Here's the drawing with two shaded views (mm, measured from the low corner). I have some questions. Round coordinates to 2 decimals unless told otherwise and drop trailing zeros. Write each loop counter-clockwise with the first axis right and the second up, starting at its lowest first coordinate (ties: lowest second). Pieces come first, ordered by that corner, then holes. Notation, with made-up numbers: M -14.5,-26.75 L -5.5,-26.75 A24 ccw -5.5,-11.75 Z; hole C 48,80 d5. An arc over 180 degrees is marked long. Use one line per item in the form item = value. Start each with the question number.
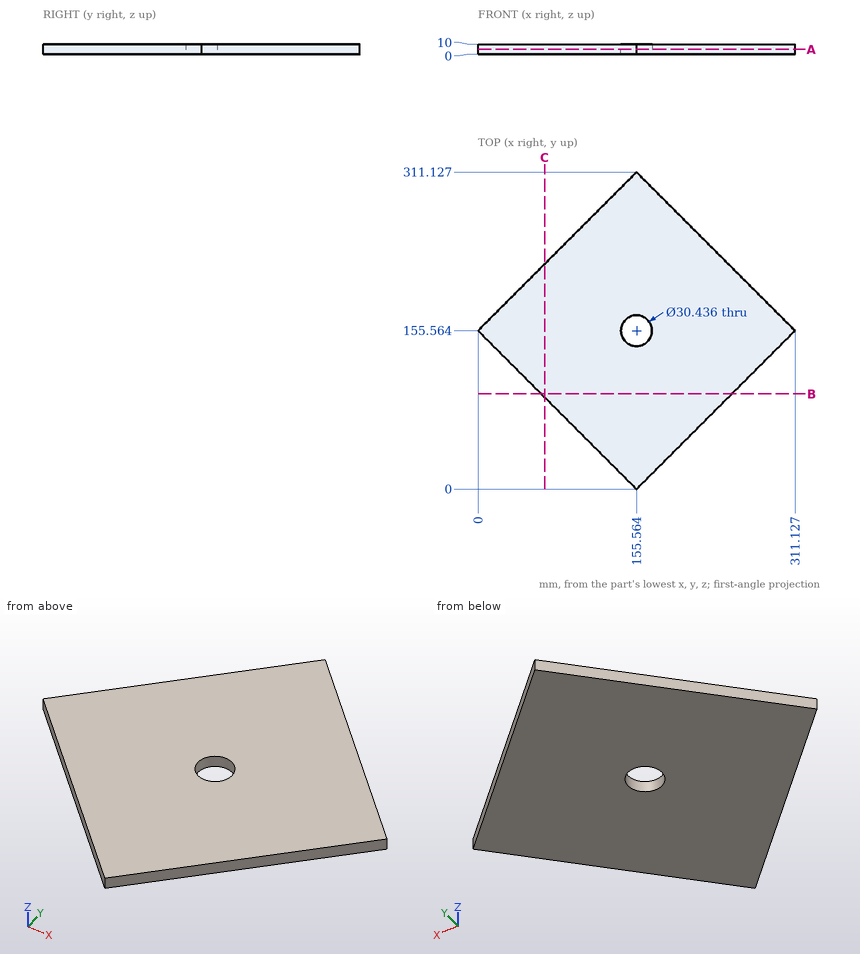
1. Please list where these lines run through material, in increasing order: line 1 along Y through (x, z) = (153.5, 7.75) (1 decimal); line 2 along Y through (x, z) = (168, 3.5) (1 decimal); line 3 along X through (y, z) = (110, 8.75) (1 decimal).
2. If we section it at B-B (y = 93.5): List the corners of the cut face in (x, z) for me.
3. If we section it at A-A (z = 4.75): List the corners of the cut face in (x, y) for me (1 decimal), and give its area (3 significant figures).
4. If we section it at C-C (x = 65.5): List the corners of the cut face in (y, z) for me, and give its area (3 significant figures).
5. Will these pins go through, and if not, where does the flat tip stop? pin 1 (6 mm diameter, centred on x = 260, z = 4.5, fed in from +Y); pin 2 (6 mm diameter, centred on y = 191.5, z = 3, fed in from -X) (1 decimal); pin 3 (1 mm diameter, centred on y = 90, z = 7, fed in from -X) (1 decimal).
Model answer:
q1.line_1 = 2.1 to 140.5, 170.6 to 309.1
q1.line_2 = 12.4 to 146.8, 164.3 to 298.7
q1.line_3 = 45.6 to 265.6
q2.outline = M 62.06,0 L 249.06,0 L 249.06,10 L 62.06,10 Z
q3.outline = M 0,155.6 L 155.6,0 L 311.1,155.6 L 155.6,311.1 Z; hole C 155.6,155.6 d30.4
q3.area = 47,700 mm2
q4.outline = M 90.06,0 L 221.06,0 L 221.06,10 L 90.06,10 Z
q4.area = 1,310 mm2
q5.pin_1 = 209.69
q5.pin_2 = 32.9
q5.pin_3 = 65.1
